Check sheet for the modelled part. Datum: model origin and axes. Units: mm. Face numbers are marked on the shaded views. A direction names the side the tool comes from. Coordinates: 2 decimals unless noted, no trailing zeros. Loops run counter-clockwise (first coordinate to the right, second up) from the corner with the lowest first, then second, coordinate; pieces in that order, holes last. Notation, with made-up numbers: M 89.5,-2 L 145.5,-2 A14 ccw 145.5,24 Z; hole C 84.25,-6.75 d2. An arc over 180 degrees is marked long. Answer as CSV lines item,"result". Start each with the question number.
from build123d import *

# Parameters (mm, degrees)
F0_R          = 12.7
F1_DEPTH      = 6.35
F0_W          = 304.8
F0_H          = 101.6
F2_DEPTH      = 6.35
F2_DEPTH_BACK = 0.0254
F3_W          = 123.825
F3_H          = 1828.8
F4_DEPTH      = 6.35
F4_DEPTH_BACK = 0.0254
F5_R          = 12.7
F6_DEPTH      = 3.175
F6_DEPTH_BACK = 3.175
F7_W          = 123.825
F7_H          = 1828.8
F8_DEPTH      = 6.35
F8_DEPTH_BACK = 0.0254
F9_W          = 304.768414
F9_H          = 101.895114
F9_R          = 12.7
F10_DEPTH     = 6.35
F12_D         = 3.175


with BuildPart() as f1:
    # F0 (on Right) → F1 (new body)
    with BuildSketch(Plane.YZ):
        Polygon((958.305541, -212.746999), (-870.494459, -212.746999), (-870.494459, -314.346999), (-752.001264, -314.346999), (-752.001264, -220.903009), (-266.81143, -220.903009), (-266.81143, -314.346999), (-266.760536, -314.346999), (958.305541, -314.346999), align=None)
        with Locations((-819.694459, -263.546999)):
            Circle(F0_R, mode=Mode.SUBTRACT)
        with Locations((704.305541, -263.546999)):
            Circle(F0_R, mode=Mode.SUBTRACT)
        with Locations((920.205541, -263.546999)):
            Circle(F0_R, mode=Mode.SUBTRACT)
        Polygon((-752.001264, -220.903009), (-752.001264, -314.346999), (-667.294459, -314.346999), (-362.494459, -314.346999), (-266.81143, -314.346999), (-266.81143, -220.903009), align=None)
    extrude(amount=-F1_DEPTH)

    # F0 (on Right) → F2 (join, two sides)
    with BuildSketch(Plane.YZ) as f2_sk:
        Polygon((-752.001264, -220.903009), (-752.001264, -314.346999), (-667.294459, -314.346999), (-362.494459, -314.346999), (-266.81143, -314.346999), (-266.81143, -220.903009), align=None)
        with BuildLine():
            Line((-667.294459, -314.346999), (-752.001264, -314.346999))
            ThreePointArc((-752.001264, -314.346999), (-716.377908, -370.75803), (-667.294459, -415.946999))
            Line((-667.294459, -415.946999), (-667.294459, -314.346999))
        make_face()
        with Locations((-514.894459, -365.146999)):
            Rectangle(F0_W, F0_H)
        with Locations((-616.494459, -377.846999)):
            Circle(F0_R, mode=Mode.SUBTRACT)
        with BuildLine():
            ThreePointArc((-362.494459, -415.946999), (-307.510614, -371.852975), (-266.760536, -314.346999))
            Line((-266.760536, -314.346999), (-266.81143, -314.346999))
            Line((-266.81143, -314.346999), (-362.494459, -314.346999))
            Line((-362.494459, -314.346999), (-362.494459, -415.946999))
        make_face()
    extrude(amount=F2_DEPTH)
    extrude(f2_sk.sketch, amount=-F2_DEPTH_BACK)

    # F3 (on face) → F4 (join, two sides)
    with BuildSketch(Plane.XY.offset(-212.746999)) as f4_sk:
        with Locations((-68.2625, 43.905541)):
            Rectangle(F3_W, F3_H)
    extrude(amount=F4_DEPTH)
    extrude(f4_sk.sketch, amount=-F4_DEPTH_BACK)

    # F5 (on face) → F6 (join, two sides)
    with BuildSketch(Plane(origin=(-130.175, 0, 0), x_dir=(0, -1, 0), z_dir=(-1, 0, 0))) as f6_sk:
        Polygon((870.494459, -314.260572), (870.494459, -212.772399), (-958.305541, -212.772399), (-958.419502, -212.772399), (-958.419502, -314.260572), align=None)
        with Locations((-920.319502, -263.516486)):
            Circle(F5_R, mode=Mode.SUBTRACT)
        with Locations((-704.419502, -263.460572)):
            Circle(F5_R, mode=Mode.SUBTRACT)
        with Locations((819.694459, -263.516486)):
            Circle(F5_R, mode=Mode.SUBTRACT)
    extrude(amount=F6_DEPTH)
    extrude(f6_sk.sketch, amount=-F6_DEPTH_BACK)

    # F7 (on face) → F8 (join, two sides)
    with BuildSketch(Plane(origin=(0, 0, -314.260572), x_dir=(1, 0, 0), z_dir=(0, 0, -1))) as f8_sk:
        with Locations((-65.0875, -43.905541)):
            Rectangle(F7_W, F7_H)
    extrude(amount=F8_DEPTH)
    extrude(f8_sk.sketch, amount=-F8_DEPTH_BACK)

    # F9 (on face) → F10 (join)
    with BuildSketch(Plane(origin=(-133.35, 0, 0), x_dir=(0, -1, 0), z_dir=(-1, 0, 0))):
        Polygon((752.8369, -221.051976), (266.6637, -221.051976), (266.6637, -314.260572), (362.727041, -314.260572), (667.495455, -314.260572), (752.8369, -314.260572), align=None)
        with BuildLine():
            Line((362.727041, -314.260572), (266.6637, -314.260572))
            ThreePointArc((266.6637, -314.260572), (307.534376, -371.959278), (362.727041, -416.155686))
            Line((362.727041, -416.155686), (362.727041, -314.260572))
        make_face()
        with Locations((515.111248, -365.208129)):
            Rectangle(F9_W, F9_H)
        with Locations((616.727041, -377.797782)):
            Circle(F9_R, mode=Mode.SUBTRACT)
        with BuildLine():
            ThreePointArc((667.495455, -416.155686), (716.949255, -370.889243), (752.8369, -314.260572))
            Line((752.8369, -314.260572), (667.495455, -314.260572))
            Line((667.495455, -314.260572), (667.495455, -416.155686))
        make_face()
    extrude(amount=F10_DEPTH)

    # F12 (through all)
    with Locations(Plane.XY.offset(-206.396999)):
        with Locations((-68.2625, 247.105541)):
            Hole(F12_D / 2)


solid = f1.part
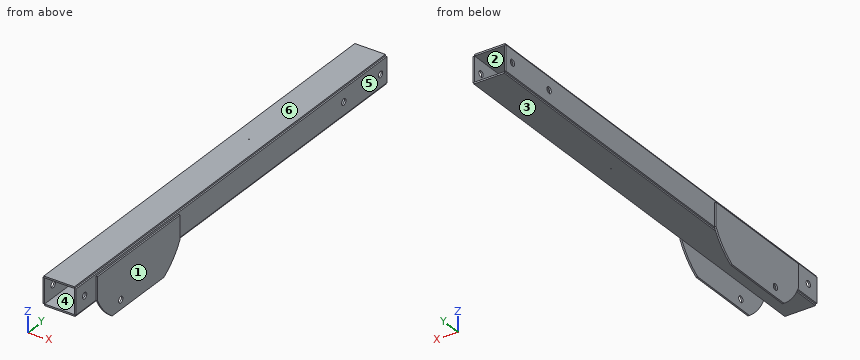
Item 1: Sectioned sample at B-B, the plane x = -108. Record the boundary of the cut face in (y, z), and give its area (3 significant figures).
Item 2: Set-up check for the marked faces 1, 2 and 3: record each of +Z, -Z, +X, -X, +Y, -Y from which the full face is reachable in a straight line by a thin tool's end or side.
Item 3: Sectioned sample at D-D, the plane y = -423. Record the boundary of the cut face in (x, z) (3 decimals).
Item 4: Release check for a two-part mould opening along Z. For the marked faces 4, 5 and 6 record: released by +Z, released by -Z, zero draft, split by the parting line, or undercut.
Item 5: Go/stop test with flat-tipped pins: pin 1 (5 mm diameter, centred on y = 454.5, z = -319, fed in from -X); pin 2 (7 mm diameter, centred on x = 4, y = -572, fed in from +Z); pin 3 (7 mm diameter, centred on y = -243.5, z = -208.5, fed in from -X) (3 decimals). Record where each tip stops, or that it passes through.
Item 6: Material ranges on line 1 (X direction, y = -680.5, z = -307); line 2 (Z direction, x = -18.5, y = -797); line 3 (X direction, y = -627.5, z = -347.5), recorded low to high. Write a range as from..to.
Item 7: Sectioned sample at C-C, the plane z = -296. Record the boundary of the cut face in (x, y), and give its area (3 significant figures).
Item 8: Sectioned sample at A-A, the plane y = -233.5. Record the boundary of the cut face in (x, z) (3 decimals).
Reply:
1,outline,"M -870.49,-320.61 L 958.31,-320.61 L 958.31,-314.24 L -870.49,-314.24 Z; M -870.49,-212.77 L 958.31,-212.77 L 958.31,-206.4 L -870.49,-206.4 Z"
1,area,"23,300 mm²"
2,face 1,"+Z, -Z, +X, +Y, -Y"
2,face 2,"+Y, -Y"
2,face 3,"-Z, +Y, -Y"
3,outline,"M -139.7,-416.156 L -133.35,-416.156 L -133.35,-314.261 L -127,-314.261 L -127,-320.611 L -3.175,-320.611 L -3.175,-314.347 L -0.025,-314.347 L -0.025,-415.947 L 6.35,-415.947 L 6.35,-220.903 L 0,-220.903 L 0,-212.747 L -6.35,-212.747 L -6.35,-206.397 L -130.175,-206.397 L -130.175,-212.772 L -133.35,-212.772 L -133.35,-221.052 L -139.7,-221.052 Z; hole M -127,-314.235 L -6.35,-314.235 L -6.35,-212.772 L -127,-212.772 Z"
4,face 4,"undercut"
4,face 5,"zero draft"
4,face 6,"released by +Z"
5,pin 1,"x = -127"
5,pin 2,"z = -220.9"
5,pin 3,"x = -130.175"
6,line 1,"-139.7..-127, -6.35..6.35"
6,line 2,"-320.61..-314.24, -212.77..-206.4"
6,line 3,"-139.7..-133.35, -0.03..6.35"
7,outline,"M -139.7,-752.84 L -133.35,-752.84 L -133.35,-870.49 L -127,-870.49 L -127,958.42 L -133.35,958.42 L -133.35,-266.66 L -139.7,-266.66 Z; M -6.35,-870.49 L 0,-870.49 L 0,-752 L 6.35,-752 L 6.35,-266.81 L 0,-266.81 L 0,958.31 L -6.35,958.31 Z"
7,area,"29,400 mm²"
8,outline,"M -133.35,-314.261 L -127,-314.261 L -127,-320.611 L -3.175,-320.611 L -3.175,-314.347 L 0,-314.347 L 0,-212.747 L -6.35,-212.747 L -6.35,-206.397 L -130.175,-206.397 L -130.175,-212.772 L -133.35,-212.772 Z; hole M -127,-314.235 L -6.35,-314.235 L -6.35,-212.772 L -127,-212.772 Z"
